Can you work these out from the model? Positions are in its coordinate system, mm. Face numbers are marked on the shaded views. Give positions to 0.01 mm unless a question says otherwise; leave off trailing zeros. Order: outer loops, then holes, each group sorted by start corner. A loop starts at its lowest first (then second) coordinate and runs counter-clockwise, first axis right, second up. Notation, with made-up numbers: (30.25, 70.25) - (55.25, 70.25) arc R22 cw to (55.25, 90.25) - close; hole circle Ø9 at (-28, 14.25). An arc over 180 degrees is marked (long way). Return JSON: item names as keys, results as strings.
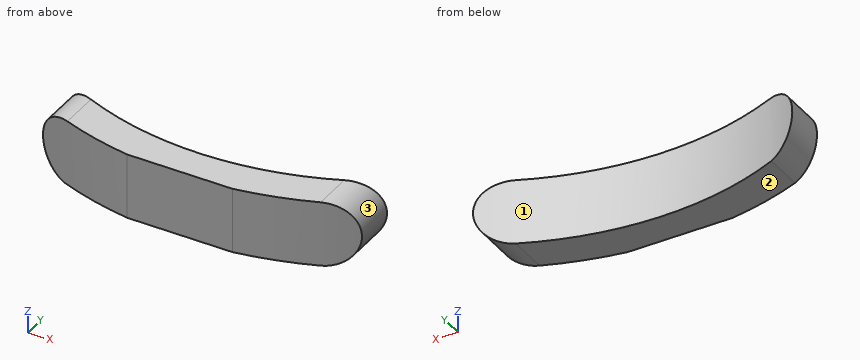
```python
from build123d import *

# Parameters (mm, degrees)
F1_DEPTH = 35
F3_DEPTH = 29.010506
F4_DEPTH = 29.010506


with BuildPart() as f1:
    # F0 (on Front) → F1 (new body)
    with BuildSketch(Plane.XZ):
        with BuildLine():
            Line((57.11247, 0), (-54.619476, 0))
            ThreePointArc((-54.619476, 0), (-69.140156, -13.855967), (-55.979297, -29.009506))
            Line((-55.979297, -29.009506), (57.11247, -29.009506))
            ThreePointArc((57.11247, -29.009506), (71.617223, -14.504753), (57.11247, 0))
        make_face()
    extrude(amount=F1_DEPTH)

    # F2 (on Top) → F3 (cut, through all)
    with BuildSketch(Plane.XY):
        with BuildLine():
            Line((102.996904, 24.844682), (-105.220917, 27.318733))
            ThreePointArc((-105.220917, 27.318733), (-1.663367, -20.32119), (102.996904, 24.844682))
        make_face()
    extrude(amount=-F3_DEPTH, mode=Mode.SUBTRACT)

    # F2 (on Top) → F4 (cut, through all)
    with BuildSketch(Plane.XY):
        with BuildLine():
            ThreePointArc((115.077005, 13.723119), (-1.858457, -36.74008), (-117.561864, 16.487342))
            Line((-117.561864, 16.487342), (-117.561864, -55.866256))
            Line((-117.561864, -55.866256), (118.521035, -63.760579))
            Line((118.521035, -63.760579), (115.077005, 13.723119))
        make_face()
    extrude(amount=-F4_DEPTH, mode=Mode.SUBTRACT)


solid = f1.part
```
1. Suppose I cut it at D-D (x = 50.5). List the corners of the cut face in (y, z) for me, plus the area to 3 significant figures.
Checks:
{"outline": "(-28.37, -29.01) - (-10.91, -29.01) - (-10.91, 0) - (-28.37, 0) - close", "area": "507 mm^2"}
2. Thinking about a two-plate mould opening in X: for the marked faces 1, 2 and 3, which applies, +X half, -X half, draft (parallel to the pull), parting line (faces both ways), or undercut?
Checks:
{"face 1": "undercut", "face 2": "draft", "face 3": "+X half"}
3. Suppose I cut it at A-A (y = -17.5). List the corners of the cut face in (x, z) for me.
Checks:
{"outline": "(-55.98, -29.01) - (-28.01, -29.01) - (-28.01, 0) - (-54.62, 0) arc R14.54 ccw to start; (28.01, -29.01) - (57.11, -29.01) arc R14.5 ccw to (57.11, 0) - (28.01, 0) - close"}
4. Suppose I cut it at C-C (z = -3). List the corners of the cut face in (x, y) for me, plus the area to 3 significant figures.
Checks:
{"outline": "(-63.46, -23.3) arc R156.42 ccw to (-23.34, -35) - (23.34, -35) arc R156.42 ccw to (65.95, -22.17) - (65.95, -3.83) arc R140 cw to (-63.46, -5.12) - close", "area": "2,140 mm^2"}
5. If I drill on L1, parallel to X at y = -9, z = -14.25; L2, parallel to X at y = -7, z = -18.75; L3, parallel to Y at x = -50, z = -18.75, over which ranges is the centre line in solid material (lowest first)? Write a range as [from, to].
Checks:
{"L1": "[-69.15, -55.18], [55.18, 71.61]", "L2": "[-68.53, -59.62], [59.62, 70.98]", "L3": "[-28.54, -11.1]"}
6. Suppose I cut it at B-B (y = -11). List the corners of the cut face in (x, z) for me, plus the area to 3 significant figures.
Checks:
{"outline": "(-55.98, -29.01) - (-50.26, -29.01) - (-50.26, 0) - (-54.62, 0) arc R14.54 ccw to start; (50.26, -29.01) - (57.11, -29.01) arc R14.5 ccw to (57.11, 0) - (50.26, 0) - close", "area": "988 mm^2"}
7. For pin 1 Ø10 at (x, z) = (14, -23) entering from +Y; pin 2 Ø3 at (x, y) = (-22.5, -23) entering from +Z; pin 3 Ø2 at (x, z) = (-5.5, -21) entering from +Y; pin 4 Ø12 at (x, z) = (30, -6) entering from +Y, each with a flat end and sliding along its axis, tell me the tip position at first contact or that it passes through.
Checks:
{"pin 1": "y = -19.04", "pin 2": "z = 0", "pin 3": "y = -20.18", "pin 4": "y = -15.62"}
